Model file for the job. Use its own axes, mm. A direction names the side the tool comes from. Coordinates: 2 decimals unless noted, no trailing zeros. Write each loop counter-clockwise with the first axis right and the second up, starting at its lowest first coordinate (ties: lowest second). Pieces come first, ordered by that corner, then holes.
Q1. Band-saw the part on B-B, the plane x = 42. Write the cut outline in (y, z).
Q2. Pull direction Z, two halves, no side cores. Call faces 1 (the flat face through (32, 100, 4)), 2 (the cylindrical face through (47.486, 113.932, -115.972)), 3 (the flat face through (35, 110, -118)), 4 (the flat face through (38, 100, -114)): released by +Z, released by -Z, zero draft, split by the parting line, or undercut.
Q3. Band-saw the part on A-A, the plane y = 113.25. Write the cut outline in (x, z).
Q4. Which spindle directions (+Z, -Z, +X, -X, +Y, -Y) get a long thin tool onto all of the face, cutting with end or side? Do faces 5 (the cylindrical face through (33.698, 119.915, -111.972)), 6 (the flat face through (35, 110, 8)). Say none if no direction does.
Q5. Band-saw the part on C-C, the plane z = -46.5. Write the cut outline in (x, y), plus the area to 3 significant figures.
Q6. Drill centre lines: probe 1 along Z at (x, y) = (36.5, 121.75); probe 2 along Y at (x, z) = (35.5, -34.5); probe 3 along X at (y, z) = (109.75, -107). Where is each one in solid material? Low to high.
Q7. Pin check, flat tips, straight feed: P1, Ø3, axis at y = 113, z = -10.5, coming from the -X side; P2, Ø1.5, axis at y = 104, z = -61, coming from the +X side. Stop position of each tip, or through.
Autodesk Inventor part; units mm, degrees
ref_plane "Work Plane2" through (-8, 0, 0) normal (0, 0, 1) x (1, 0, 0)
ref_plane "YZ Plane" through (0, 0, 0) normal (1, 0, 0) x (0, 1, 0)
ref_plane "XZ Plane" through (0, 0, 0) normal (0, 1, 0) x (-1, 0, 0)
ref_plane "Work Plane1" through (70, 0, -110) normal (0, 0, -1) x (-1, 0, 0)
sketch "Sketch1" plane through (70, 0, -110) normal (0, 0, -1) x (-1, 0, 0)
  circle A0 centre (35, 110) radius 13.5
  circle A1 centre (35, 110) radius 13.09
  point P0 (70, 0)
  dimension "d2" = 0.41
ref_plane "Work Plane2" through (-8, 0, 0) normal (0, 0, 1) x (1, 0, 0)
extrude "Extrusion1" add sketch "Sketch1" against normal up to surface (110 mm away) contours A1
sketch "Sketch2" plane through (35, 110, 0) normal (0, 0, 1) x (1, 0, 0)
  circle A0 centre (0, 0) radius 13.09
  circle A1 centre (0, 0) radius 10
  point P0 (-35, -110)
  dimension "d3" = 20
extrude "Extrusion2" add sketch "Sketch2" along normal blind 4 contours A1
sketch "Sketch3" plane through (35, 110, 4) normal (0, 0, 1) x (1, 0, 0)
  circle A0 centre (0, 0) radius 13.09
  point P0 (-35, -110)
extrude "Extrusion3" add sketch "Sketch3" along normal blind 4
ref_plane "Work Plane3" through (35, 110, -55) normal (0, 0, 1) x (1, 0, 0)
mirror "Mirror1" about plane through (35, 110, -55) normal (0, 0, 1) of "Extrusion2", "Extrusion3"
equation "\"BendRadius\" = Thickness"
equation "\"BendReliefWidth\" = Thickness"
equation "\"BendReliefDepth\" = 0.5 * Thickness"
equation "\"CornerReliefSize\" = 4 * Thickness"
equation "\"MinimumRemnant\" = 2 * Thickness"
equation "\"TransitionRadius\" = BendRadius"
equation "\"JacobiRadiusSize\" = BendRadius"
equation "\"GapSize\" = Thickness"
properties part number "axle_3DPrint"
Answer sheet:
1. outline: (98.94, -118) - (121.06, -118) - (121.06, -114) - (117.14, -114) - (117.14, -110) - (121.06, -110) - (121.06, 0) - (117.14, 0) - (117.14, 4) - (121.06, 4) - (121.06, 8) - (98.94, 8) - (98.94, 4) - (102.86, 4) - (102.86, 0) - (98.94, 0) - (98.94, -110) - (102.86, -110) - (102.86, -114) - (98.94, -114) - close
2. face 1: undercut
2. face 2: zero draft
2. face 3: released by -Z
2. face 4: undercut
3. outline: (22.32, -118) - (47.68, -118) - (47.68, -114) - (44.46, -114) - (44.46, -110) - (47.68, -110) - (47.68, 0) - (44.46, 0) - (44.46, 4) - (47.68, 4) - (47.68, 8) - (22.32, 8) - (22.32, 4) - (25.54, 4) - (25.54, 0) - (22.32, 0) - (22.32, -110) - (25.54, -110) - (25.54, -114) - (22.32, -114) - close
4. face 5: none
4. face 6: +Z, +X, -X, +Y, -Y
5. outline: circle Ø26.18 at (35, 110)
5. area: 538 mm2
6. probe 1: z = -118 to -114, -110 to 0, 4 to 8
6. probe 2: y = 96.92 to 123.08
6. probe 3: x = 21.91 to 48.09
7. P1: stops at x = 22
7. P2: stops at x = 46.99
